The listing builds one solid part. Answer for the finished solid, in the listing's coordinates (mm). Round coordinates to 2 decimals unless told otherwise and drop trailing zeros. Write each loop counter-clockwise with the first axis right and the second up, starting at its lowest first coordinate (ties: lowest second). Pieces come first, ordered by that corner, then holes. Notation, with made-up numbers: M 40.25,27.5 L 93.25,27.5 A14 ccw 93.25,50.5 Z; hole C 20,56.5 d7. An arc over 180 degrees is marked long. Answer as CSV lines item,"result". Start each with the question number.
from build123d import *

# Parameters (mm, degrees)
SKETCH1_W           = 60
SKETCH1_H           = 110
SKETCH1_R           = 2.5
BOSS_EXTRUDE1_DEPTH = 5


with BuildPart() as part:
    # Sketch1 → Boss-Extrude1 (new body)
    with BuildSketch(Plane.XY):
        with Locations((30, -55)):
            Rectangle(SKETCH1_W, SKETCH1_H)
        with Locations((8.879726404, -15)):
            Circle(SKETCH1_R, mode=Mode.SUBTRACT)
        with Locations((49.096380092, -15)):
            Circle(SKETCH1_R, mode=Mode.SUBTRACT)
        with Locations((49.743242135, -43.54)):
            Circle(SKETCH1_R, mode=Mode.SUBTRACT)
        with Locations((8.252207519, -43.54)):
            Circle(SKETCH1_R, mode=Mode.SUBTRACT)
        with Locations((7, -100)):
            Circle(SKETCH1_R, mode=Mode.SUBTRACT)
        with Locations(Location((53, -100, 0), (0, 0, 180))):
            Circle(SKETCH1_R, mode=Mode.SUBTRACT)
    extrude(amount=BOSS_EXTRUDE1_DEPTH)


solid = part.part
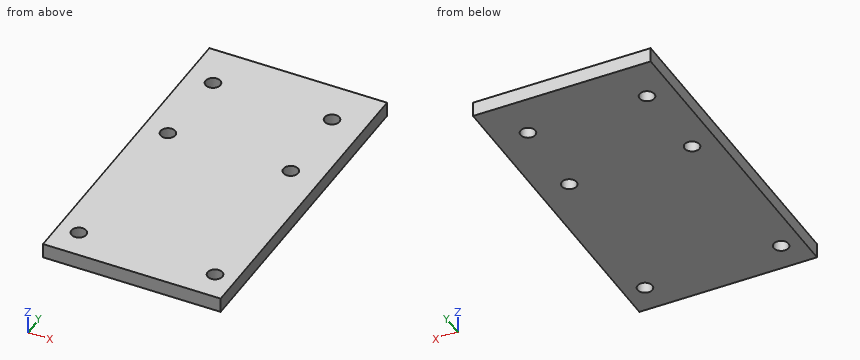
Q1. Find section A-A (y = -100). Determine the outline of the cut face in (x, z), plus the area to 3 significant figures.
Q2. Straight lines are drawn through the part: L1, parallel to Y at x = 53, z = 2.95; L2, parallel to Y at x = 6, z = 1.05; L3, parallel to Y at x = 7.5, z = 2.1. For each, find the intervals that lie inside material, in ascending order.
Q3. Find section B-B (z = 3.4). Determine the outline of the cut face in (x, y), plus the area to 3 significant figures.
Q4. Each of these flat-tipped pins is pushed along its axis until it touches: P1, Ø4.5, axis at x = 53, y = -100, coming from the -Z side; P2, Ø6, axis at x = 8.25, y = -43.54, coming from the +Z side. Where does it stop, or does it pass through?
Q5. Find section C-C (x = 8). Determine the outline of the cut face in (y, z).
Reported:
1,outline,"M 0,0 L 4.5,0 L 4.5,5 L 0,5 Z; M 9.5,0 L 50.5,0 L 50.5,5 L 9.5,5 Z; M 55.5,0 L 60,0 L 60,5 L 55.5,5 Z"
1,area,"250 mm2"
2,L1,"y = -110 to -102.5, -97.5 to 0"
2,L2,"y = -110 to -102.29, -97.71 to -44.63, -42.45 to 0"
2,L3,"y = -110 to -102.45, -97.55 to -45.92, -41.16 to -17.08, -12.92 to 0"
3,outline,"M 0,-110 L 60,-110 L 60,0 L 0,0 Z; hole C 7,-100 d5; hole C 8.25,-43.54 d5; hole C 8.88,-15 d5; hole C 49.1,-15 d5; hole C 49.74,-43.54 d5; hole C 53,-100 d5"
3,area,"6,480 mm2"
4,P1,"passes through"
4,P2,"stops at z = 5"
5,outline,"M -110,0 L -102.29,0 L -102.29,5 L -110,5 Z; M -97.71,0 L -46.03,0 L -46.03,5 L -97.71,5 Z; M -41.05,0 L -17.34,0 L -17.34,5 L -41.05,5 Z; M -12.66,0 L 0,0 L 0,5 L -12.66,5 Z"
